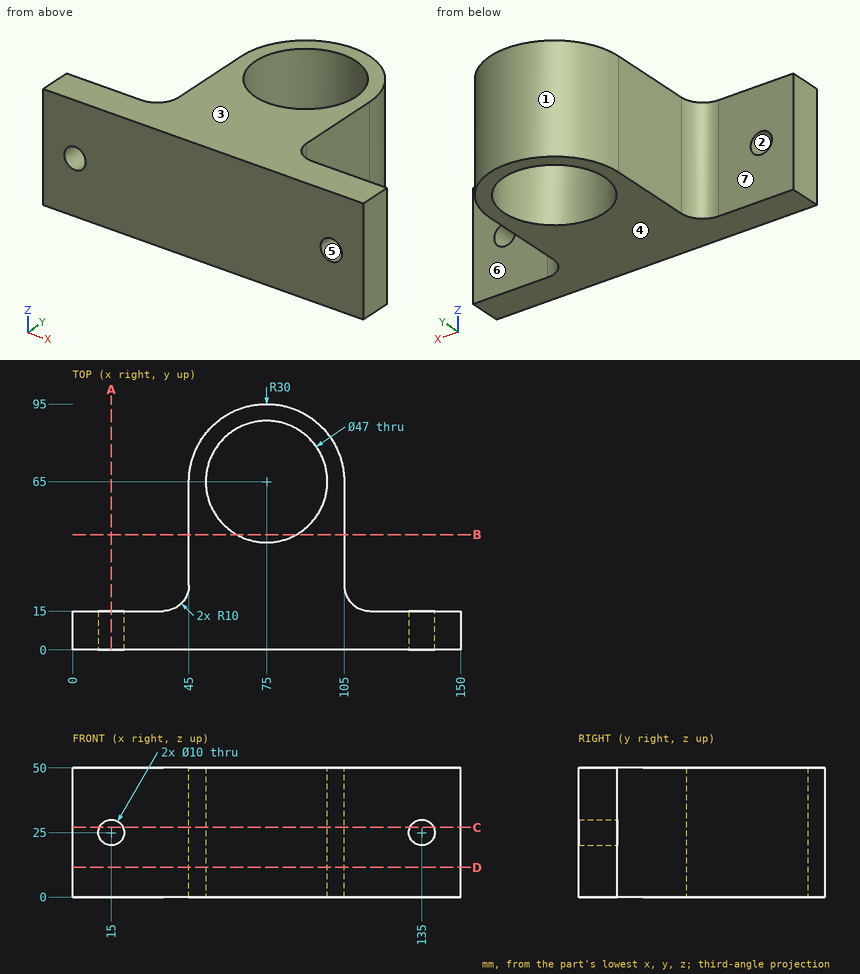
Can you work these out from the drawing? Everything is in mm from the part's minimum corner. A direction names the side the tool comes from. Coordinates: 2 decimals unless noted, no trailing zeros. Loops run counter-clockwise (first coordinate to the right, second up) from the corner with the lowest first, then second, coordinate; pieces in that order, holes last.
1) Thinking about a two-plate mould opening in Z: for the marked faces 1, 2, 3 and 4, which applies, released by +Z, released by -Z, zero draft, split by the parting line, or undercut?
Reported:
face 1: zero draft
face 2: undercut
face 3: released by +Z
face 4: released by -Z
2) Imagine slicing it at C-C (z = 27). List the corners of the cut face in (x, y) for me.
Reported:
outline: (0, 0) - (10.42, 0) - (10.42, 15) - (0, 15) - close; (19.58, 0) - (130.42, 0) - (130.42, 15) - (115, 15) arc R10 cw to (105, 25) - (105, 65) arc R30 ccw to (45, 65) - (45, 25) arc R10 cw to (35, 15) - (19.58, 15) - close; (139.58, 0) - (150, 0) - (150, 15) - (139.58, 15) - close; hole circle Ø47 at (75, 65)
3) Will these pins go through, and if not, where does the flat tip stop? pin 1 Ø11.5 at (x, z) = (135, 25) entering from +Y; pin 2 Ø8 at (y, z) = (71, 9.5) entering from +X; pin 3 Ø12 at (y, z) = (12, 44.5) entering from -X; pin 4 Ø1 at (y, z) = (59, 24.5) entering from +X.
Reported:
pin 1: stops at y = 15
pin 2: stops at x = 104.93
pin 3: stops at x = 0
pin 4: stops at x = 105
4) Imagine slicing it at D-D (z = 11.5). List the corners of the cut face in (x, y) for me, and give its area (3 significant figures).
Reported:
outline: (0, 0) - (150, 0) - (150, 15) - (115, 15) arc R10 cw to (105, 25) - (105, 65) arc R30 ccw to (45, 65) - (45, 25) arc R10 cw to (35, 15) - (0, 15) - close; hole circle Ø47 at (75, 65)
area: 4,970 mm2
5) Imagine slicing it at B-B (y = 44.5). List the corners of the cut face in (x, z) for me.
Reported:
outline: (45, 0) - (63.51, 0) - (63.51, 50) - (45, 50) - close; (86.49, 0) - (105, 0) - (105, 50) - (86.49, 50) - close
6) Which directions (+Z, -Z, +X, -X, +Y, -Y) give clear straight access to the entire face, cutting with the end or side of a thin tool? Please do the marked faces 5, 6 and 7.
Reported:
face 5: +Y, -Y
face 6: +Z, -Z, +X, +Y
face 7: +Z, -Z, -X, +Y
7) Imagine slicing it at A-A (x = 15). List the corners of the cut face in (y, z) for me, and give its area (3 significant figures).
Reported:
outline: (0, 0) - (15, 0) - (15, 20) - (0, 20) - close; (0, 30) - (15, 30) - (15, 50) - (0, 50) - close
area: 600 mm2
8) Please list where these lines run through material, in increasing order: line 1 along Y through (x, z) = (75, 28.5); line 2 along Z through (x, y) = (15, 5); line 3 along Y through (x, z) = (125.5, 37.5).
Reported:
line 1: y = 0 to 41.5, 88.5 to 95
line 2: z = 0 to 20, 30 to 50
line 3: y = 0 to 15
